```python
from build123d import *

# Parameters (mm, degrees)
SKETCH1_R               = 9.25
BOSS_EXTRUDE1_DEPTH     = 10
SKETCH2_R               = 10
BOSS_EXTRUDE2_DEPTH     = 10
SKETCH3_W               = 12
SKETCH3_H               = 16
BOSS_EXTRUDE3_DEPTH     = 20
CUT_EXTRUDE1_DEPTH      = 5
CUT_EXTRUDE1_DEPTH_BACK = 30
SKETCH4_3_R             = 6
CUT_EXTRUDE2_DEPTH      = 17
SKETCH5_W               = 6
SKETCH5_H               = 20
CUT_EXTRUDE3_DEPTH      = 19


with BuildPart() as part:
    # Sketch1 → Boss-Extrude1 (new body)
    with BuildSketch(Plane.XY):
        Circle(SKETCH1_R)
    extrude(amount=BOSS_EXTRUDE1_DEPTH)

    # Sketch2 → Boss-Extrude2 (add)
    with BuildSketch(Plane(origin=(0, 0, 0), x_dir=(-1, 0, 0), z_dir=(0, 0, -1))):
        Circle(SKETCH2_R)
    extrude(amount=BOSS_EXTRUDE2_DEPTH)

    # Sketch3 → Boss-Extrude3 (add)
    with BuildSketch(Plane(origin=(0, 0, -10), x_dir=(-1, 0, 0), z_dir=(0, 0, -1))):
        Rectangle(SKETCH3_W, SKETCH3_H)
    extrude(amount=BOSS_EXTRUDE3_DEPTH)

    # Sketch4 → Cut-Extrude1 (cut, two sides)
    with BuildSketch(Plane(origin=(6, 0, 0), x_dir=(0, 0, -1), z_dir=(1, 0, 0))) as cut_extrude1_sk:
        with BuildLine():
            Line((30, 8), (22, 8))
            ThreePointArc((22, 8), (27.656854249, 5.656854249), (30, 0))
            Line((30, 0), (30, 8))
        make_face()
        with BuildLine():
            Line((30, -8), (30, 0))
            ThreePointArc((30, 0), (27.656854249, -5.656854249), (22, -8))
            Line((22, -8), (30, -8))
        make_face()
    extrude(amount=CUT_EXTRUDE1_DEPTH, mode=Mode.SUBTRACT)
    extrude(cut_extrude1_sk.sketch, amount=-CUT_EXTRUDE1_DEPTH_BACK, mode=Mode.SUBTRACT)

    # Sketch4<3> → Cut-Extrude2 (cut, through all)
    with BuildSketch(Plane(origin=(6, 0, 0), x_dir=(0, 0, -1), z_dir=(1, 0, 0))):
        with Locations((22, 0)):
            Circle(SKETCH4_3_R)
    extrude(amount=-CUT_EXTRUDE2_DEPTH, mode=Mode.SUBTRACT)

    # Sketch5 → Cut-Extrude3 (cut, through all)
    with BuildSketch(Plane(origin=(0, 8, 0), x_dir=(1, 0, 0), z_dir=(0, 1, 0))):
        with Locations((-3, 20)):
            Rectangle(SKETCH5_W, SKETCH5_H)
    extrude(amount=-CUT_EXTRUDE3_DEPTH, mode=Mode.SUBTRACT)


solid = part.part
```
Design review of the part built by this model. Coordinates are the model's own, in mm. A direction names the side the tool comes from. Give positions to 0.01 mm unless a question says otherwise; leave off trailing zeros. Loops run counter-clockwise (first coordinate to the right, second up) from the corner with the lowest first, then second, coordinate; pieces in that order, holes last. Notation, with made-up numbers: (-24.75, 71.5) -> (-2.75, 71.5) arc R21 cw to (-2.75, 83.5) -> close; hole circle Ø7 at (63, 22.5). An arc over 180 degrees is marked (long way). One line per item, written item: value.
Q1. For pin 1 Ø5 at (y, z) = (-0.5, -16.5) entering from -X; pin 2 Ø5 at (y, z) = (2, -15) entering from +X; pin 3 Ø1.2 at (x, y) = (7.5, -1) entering from -Z, all flat-tipped, find the tip position at first contact; note any pin that passes through.
Numbers:
pin 1: stops at x = 0
pin 2: stops at x = 6
pin 3: stops at z = -10
Q2. We need section A-A on y = 1.5. Give the boundary of the cut face in (x, z).
Numbers:
outline: (-9.89, -10) -> (0, -10) -> (0, -16.19) -> (6, -16.19) -> (6, -10) -> (9.89, -10) -> (9.89, 0) -> (9.13, 0) -> (9.13, 10) -> (-9.13, 10) -> (-9.13, 0) -> (-9.89, 0) -> close; (0, -29.86) -> (6, -29.86) -> (6, -27.81) -> (0, -27.81) -> close
Q3. Machinability: for faces 4 (the cylindrical face through (-2.01, -9.03, 4.93)), 5 (the flat face through (6, 0, -15)), 6 (the flat face through (3, -8, -16)), 7 (the flat face through (3, 8, -16)), which of the approach directions +Z, -Z, +X, -X, +Y, -Y give a long, thin tool a straight path to every point of the face, cutting with its end or side? Answer none if there is none.
Numbers:
face 4: +Z
face 5: -Z, +X, +Y, -Y
face 6: -Z, +X, -X, -Y
face 7: -Z, +X, -X, +Y
Q4. For L1, parallel to X at y = 0.25, z = -9; L2, parallel to Y at x = 3.45, z = -22, list the stretches that pass through material, from the lowest coordinate up.
Numbers:
L1: x = -10 to 10
L2: y = -8 to -6, 6 to 8
Q5. We need section D-D on y = -1. Give the boundary of the cut face in (x, z), and give its area (3 significant figures).
Numbers:
outline: (-9.95, -10) -> (0, -10) -> (0, -16.08) -> (6, -16.08) -> (6, -10) -> (9.95, -10) -> (9.95, 0) -> (9.2, 0) -> (9.2, 10) -> (-9.2, 10) -> (-9.2, 0) -> (-9.95, 0) -> close; (0, -29.94) -> (6, -29.94) -> (6, -27.92) -> (0, -27.92) -> close
area: 432 mm^2
Q6. We need section B-B on z = -13. Give the boundary of the cut face in (x, y).
Numbers:
outline: (0, -8) -> (6, -8) -> (6, 8) -> (0, 8) -> close
Q7. Draft analysis for pull direction Z (two halves, no side actions). For faces 1 (the cylindrical face through (3.04, -3.65, -17.24)), 2 (the flat face through (0, 0, -15)), 3 (the flat face through (-3, -9, 0)), state which applies: pulls with the +Z half, pulls with the -Z half, needs draft (parallel to the pull), parting line crosses it, or undercut.
Numbers:
face 1: undercut
face 2: needs draft
face 3: pulls with the +Z half
Q8. We need section C-C on x = -5.5. Give the boundary of the cut face in (y, z).
Numbers:
outline: (-8.35, -10) -> (8.35, -10) -> (8.35, 0) -> (7.44, 0) -> (7.44, 10) -> (-7.44, 10) -> (-7.44, 0) -> (-8.35, 0) -> close
